from build123d import *

# Parameters (mm, degrees)
BOSS_EXTRUDE2_DEPTH      = 3.048
SKETCH4_R                = 38.1
CUT_EXTRUDE3_DEPTH       = 4.048
BOSS_EXTRUDE3_DEPTH      = 3.175
SKETCH12_R               = 1.143
CUT_EXTRUDE9_DEPTH       = 4.175
SKETCH15_R               = 1.651
CUT_EXTRUDE12_DEPTH      = 75.692
SKETCH17_R               = 1.651
CUT_EXTRUDE14_DEPTH      = 97.79
SKETCH18_R               = 12.192
CUT_EXTRUDE15_DEPTH      = 35.56
SKETCH19_R               = 3.175
CUT_EXTRUDE16_DEPTH      = 103.378
CUT_EXTRUDE16_DEPTH_BACK = 48.768
SKETCH5_R                = 12.192
CUT_EXTRUDE6_DEPTH       = 4.175
FILLET1_R                = 2.54


with BuildPart() as part:
    # Sketch1 → Boss-Extrude2 (new body)
    with BuildSketch(Plane.XY):
        with BuildLine():
            Line((-60.107370596, 33.02), (-55.027370596, 33.02))
            Line((-55.027370596, 33.02), (-55.027370596, -33.02))
            Line((-55.027370596, -33.02), (-60.107370596, -33.02))
            ThreePointArc((-60.107370596, -33.02), (0, -68.58), (60.107370596, -33.02))
            Line((60.107370596, -33.02), (55.027370596, -33.02))
            Line((55.027370596, -33.02), (55.027370596, 33.02))
            Line((55.027370596, 33.02), (60.107370596, 33.02))
            ThreePointArc((60.107370596, 33.02), (0, 68.58), (-60.107370596, 33.02))
        make_face()
    extrude(amount=BOSS_EXTRUDE2_DEPTH)

    # Sketch4 → Cut-Extrude3 (cut, through all)
    with BuildSketch(Plane(origin=(0, 0, 0), x_dir=(-1, 0, 0), z_dir=(0, 0, -1))):
        with Locations((0, -86.312058398)):
            Circle(SKETCH4_R)
    extrude(amount=-CUT_EXTRUDE3_DEPTH, mode=Mode.SUBTRACT)

    # Sketch9 → Boss-Extrude3 (add)
    with BuildSketch(Plane(origin=(0, 0, 0), x_dir=(-1, 0, 0), z_dir=(0, 0, -1))):
        with BuildLine():
            Line((12.7, 67.39381574), (0, 75))
            Line((0, 75), (-12.7, 67.39381574))
            ThreePointArc((-12.7, 67.39381574), (0, 68.58), (12.7, 67.39381574))
        make_face()
    extrude(amount=-BOSS_EXTRUDE3_DEPTH)

    # Sketch12 → Cut-Extrude9 (cut, through all)
    with BuildSketch(Plane(origin=(0, 0, 0), x_dir=(-1, 0, 0), z_dir=(0, 0, -1))):
        with Locations((6.731, 62.23)):
            Circle(SKETCH12_R)
        with Locations((-6.731, 62.23)):
            Circle(SKETCH12_R)
    extrude(amount=-CUT_EXTRUDE9_DEPTH, mode=Mode.SUBTRACT)

    # Sketch15 → Cut-Extrude12 (cut)
    with BuildSketch(Plane(origin=(30.092005081, 4.08352975, -3.048), x_dir=(-1, 0, 0), z_dir=(0, 0, -1))):
        with Locations((63.757223581, 17.50647025)):
            Circle(SKETCH15_R)
        with Locations((63.757223581, -25.67352975)):
            Circle(SKETCH15_R)
        with Locations((-3.552776419, -25.67352975)):
            Circle(SKETCH15_R)
        with Locations((-3.552776419, 17.50647025)):
            Circle(SKETCH15_R)
    extrude(amount=-CUT_EXTRUDE12_DEPTH, mode=Mode.SUBTRACT)

    # Sketch17 → Cut-Extrude14 (cut)
    with BuildSketch(Plane(origin=(30.092005081, 4.08352975, -33.0835), x_dir=(-1, 0, 0), z_dir=(0, 0, -1))):
        with Locations((4.154396091, -49.728759131)):
            Circle(SKETCH17_R)
        with Locations((56.02961407, -49.728759131)):
            Circle(SKETCH17_R)
        with Locations((4.154396091, 41.38247025)):
            Circle(SKETCH17_R)
        with Locations((56.02961407, 41.38247025)):
            Circle(SKETCH17_R)
    extrude(amount=-CUT_EXTRUDE14_DEPTH, mode=Mode.SUBTRACT)

    # Sketch18 → Cut-Extrude15 (cut)
    with BuildSketch(Plane(origin=(0, 0, 0), x_dir=(-1, 0, 0), z_dir=(0, 0, -1))):
        with Locations((31.75, 0)):
            Circle(SKETCH18_R)
        with Locations((-31.75, 0)):
            Circle(SKETCH18_R)
    extrude(amount=-CUT_EXTRUDE15_DEPTH, mode=Mode.SUBTRACT)

    # Sketch19 → Cut-Extrude16 (cut, two sides)
    with BuildSketch(Plane(origin=(30.092005081, 4.08352975, 3.048), x_dir=(-1, 0, 0), z_dir=(0, 0, -1))) as cut_extrude16_sk:
        with Locations((-16.897994919, 21.31647025)):
            Circle(SKETCH19_R)
        with Locations((77.082005081, 21.31647025)):
            Circle(SKETCH19_R)
        with Locations((30.092005081, 21.31647025)):
            Circle(SKETCH19_R)
        with Locations((77.082005081, -29.48352975)):
            Circle(SKETCH19_R)
        with Locations((30.092005081, -29.48352975)):
            Circle(SKETCH19_R)
        with Locations((-16.897994919, -29.48352975)):
            Circle(SKETCH19_R)
    extrude(amount=CUT_EXTRUDE16_DEPTH, mode=Mode.SUBTRACT)
    extrude(cut_extrude16_sk.sketch, amount=-CUT_EXTRUDE16_DEPTH_BACK, mode=Mode.SUBTRACT)

    # Sketch5 → Cut-Extrude6 (cut, through all)
    with BuildSketch(Plane(origin=(0, 0, 0), x_dir=(-1, 0, 0), z_dir=(0, 0, -1))):
        with BuildLine():
            Line((45.125787008, -51.860979099), (48.493383054, -48.493383054))
            Line((48.493383054, -48.493383054), (33.244765274, -33.244765274))
            Line((33.244765274, -33.244765274), (15.887580142, -16.296407899))
            ThreePointArc((15.887580142, -16.296407899), (15.502857332, -15.608744759), (15.036339126, -14.973722712))
            ThreePointArc((15.036339126, -14.973722712), (14.151046139, -13.510927072), (12.484618985, -13.128127778))
            ThreePointArc((12.484618985, -13.128127778), (4.300657145, -21.652046912), (16.112224352, -21.303752637))
            Line((16.112224352, -21.303752637), (29.410338797, -36.145530887))
            Line((29.410338797, -36.145530887), (45.125787008, -51.860979099))
        make_face()
        with BuildLine():
            ThreePointArc((15.036339126, 14.973722712), (15.502857332, 15.608744759), (15.887580142, 16.296407899))
            Line((15.887580142, 16.296407899), (33.244765274, 33.244765274))
            Line((33.244765274, 33.244765274), (48.493383054, 48.493383054))
            Line((48.493383054, 48.493383054), (45.125787008, 51.860979099))
            Line((45.125787008, 51.860979099), (29.410338797, 36.145530887))
            Line((29.410338797, 36.145530887), (16.112224352, 21.303752637))
            ThreePointArc((16.112224352, 21.303752637), (4.300657145, 21.652046912), (12.484618985, 13.128127778))
            ThreePointArc((12.484618985, 13.128127778), (14.151046139, 13.510927072), (15.036339126, 14.973722712))
        make_face()
        with BuildLine():
            ThreePointArc((-12.484618985, 13.128127778), (-4.300657145, 21.652046912), (-16.112224352, 21.303752637))
            Line((-16.112224352, 21.303752637), (-29.410338797, 36.145530887))
            Line((-29.410338797, 36.145530887), (-45.125787008, 51.860979099))
            Line((-45.125787008, 51.860979099), (-48.493383054, 48.493383054))
            Line((-48.493383054, 48.493383054), (-33.244765274, 33.244765274))
            Line((-33.244765274, 33.244765274), (-15.887580142, 16.296407899))
            ThreePointArc((-15.887580142, 16.296407899), (-15.502857332, 15.608744759), (-15.036339126, 14.973722712))
            ThreePointArc((-15.036339126, 14.973722712), (-14.151046139, 13.510927072), (-12.484618985, 13.128127778))
        make_face()
        with BuildLine():
            Line((-45.125787008, -51.860979099), (-29.410338797, -36.145530887))
            Line((-29.410338797, -36.145530887), (-16.112224352, -21.303752637))
            ThreePointArc((-16.112224352, -21.303752637), (-4.300657145, -21.652046912), (-12.484618985, -13.128127778))
            ThreePointArc((-12.484618985, -13.128127778), (-14.151046139, -13.510927072), (-15.036339126, -14.973722712))
            ThreePointArc((-15.036339126, -14.973722712), (-15.502857332, -15.608744759), (-15.887580142, -16.296407899))
            Line((-15.887580142, -16.296407899), (-33.244765274, -33.244765274))
            Line((-33.244765274, -33.244765274), (-48.493383054, -48.493383054))
            Line((-48.493383054, -48.493383054), (-45.125787008, -51.860979099))
        make_face()
        Circle(SKETCH5_R)
        with Locations((0, 44.45)):
            Circle(SKETCH5_R)
    extrude(amount=-CUT_EXTRUDE6_DEPTH, mode=Mode.SUBTRACT)

    # Fillet1
    fillet1_edges = [part.edges().sort_by_distance(p)[0] for p in [
        (-16.112224352, -21.303752637, 1.524),
        (-16.112224352, 21.303752637, 1.524),
        (16.112224352, 21.303752637, 1.524),
        (16.112224352, -21.303752637, 1.524),
    ]]
    fillet(fillet1_edges, radius=FILLET1_R)


solid = part.part
Here's how the part is built. I have some questions about the finished solid (model axes, mm). A direction names the side the tool comes from. Coordinates: 2 decimals unless noted, no trailing zeros. Loops run counter-clockwise (first coordinate to the right, second up) from the corner with the lowest first, then second, coordinate; pieces in that order, holes last.
1. Imagine slicing it at C-C, the plane x = -47. Please give me the cut outline in (y, z).
2. Imagine slicing it at D-D, the plane y = -7.5. Please give me the cut outline in (x, z), and give its area (3 significant figures).
3. Imagine slicing it at A-A, the plane x = 46.99. Please give me the cut outline in (y, z) (3 decimals), and give its area (3 significant figures).
4. Imagine slicing it at B-B, the plane y = 8. Please give me the cut outline in (x, z).
5. If we mould it in two halves opening along X, with no side actions, what happens to faces 1 (the flat face through (37.319, -44.054, 1.503)), 2 (the flat face through (58, -33.02, 2)), 3 (the flat face through (6.26, 71.25, 1.57))? For each: pulls with the +X half, pulls with the -X half, needs draft (parallel to the pull), parting line crosses it, or undercut.
6. I need wall thicknesses on L1, parallel to Y at x = 0, z = 2.25 (3 decimals); L2, parallel to X at y = 62, z = 2.65; L3, parallel to Y at x = -5.5, z = 2.3. Which ranges of each line are inside material? Lowest first, please.
7. For P1, Ø1.5, axis at x = 34.5, z = 1.5, coming from the +Y side; P2, Ø10, axis at x = -10.14, y = -19.06, coming from the -Z side; P3, Ø7.5, axis at x = -46.99, y = 25.4, coming from the +Z side; P4, Ø1.5, axis at x = -57, z = 1, coming from the +Y side, each with a flat end and sliding along its axis, tell me the tip position at first contact or that it passes through.
8. For faces 4 (the cylindrical face through (-37.63, -57.334, 1.503)), 5 (the flat face through (41, -41, 2)), 6 (the flat face through (-55.027, 0, 2)), which set-ups out of +Z, -Z, +X, -X, +Y, -Y let a thin tool reach every point of the face, with its end or its side?
Taken from the geometry:
1. outline: (-47, 0) - (-28.57, 0) - (-28.57, 3.05) - (-47, 3.05) - close; (-22.23, 0) - (22.23, 0) - (22.23, 3.05) - (-22.23, 3.05) - close; (28.57, 0) - (47, 0) - (47, 3.05) - (28.57, 3.05) - close
2. outline: (-55.03, 0) - (-41.36, 0) - (-41.36, 3.05) - (-55.03, 3.05) - close; (-22.14, 0) - (-9.61, 0) - (-9.61, 3.05) - (-22.14, 3.05) - close; (9.61, 0) - (22.14, 0) - (22.14, 3.05) - (9.61, 3.05) - close; (41.36, 0) - (55.03, 0) - (55.03, 3.05) - (41.36, 3.05) - close
2. area: 160 mm2
3. outline: (-46.99, 0) - (-28.575, 0) - (-28.575, 3.048) - (-46.99, 3.048) - close; (-22.225, 0) - (22.225, 0) - (22.225, 3.048) - (-22.225, 3.048) - close; (28.575, 0) - (46.99, 0) - (46.99, 3.048) - (28.575, 3.048) - close
3. area: 248 mm2
4. outline: (-55.03, 0) - (-40.95, 0) - (-40.95, 3.05) - (-55.03, 3.05) - close; (-22.55, 0) - (-9.2, 0) - (-9.2, 3.05) - (-22.55, 3.05) - close; (9.2, 0) - (22.55, 0) - (22.55, 3.05) - (9.2, 3.05) - close; (40.95, 0) - (55.03, 0) - (55.03, 3.05) - (40.95, 3.05) - close
5. face 1: undercut
5. face 2: needs draft
5. face 3: pulls with the +X half
6. L1: y = -48.212 to -28.575, -22.225 to -12.192, 12.192 to 22.225, 28.575 to 32.258, 56.642 to 75
6. L2: x = -29.31 to -7.85, -5.61 to 5.61, 7.85 to 29.31
6. L3: y = -48.61 to -23.45, -14.67 to -10.88, 10.88 to 14.67, 23.45 to 33.57, 55.33 to 71.71
7. P1: stops at y = 59.7
7. P2: passes through
7. P3: stops at z = 3.05
7. P4: stops at y = 39.23
8. face 4: +Z, -Z, -X, -Y
8. face 5: +Z, -Z
8. face 6: +Z, -Z, -X
